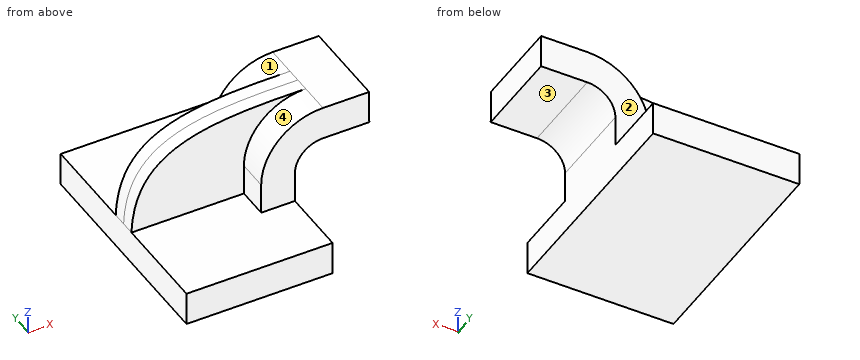
```python
from build123d import *

# Parameters (mm, degrees)
F1_DEPTH = 63.5
F2_DEPTH = 25.4
F3_DEPTH = 7.9375


with BuildPart() as f1:
    # F0 (on Front) → F1 (new body, symmetric)
    with BuildSketch(Plane.XZ):
        Polygon((22.225, 9.525), (-41.275, 9.525), (-41.275, -9.525), (41.275, -9.525), (41.275, 9.525), align=None)
    extrude(amount=F1_DEPTH, both=True)

    # F0 (on Front) → F2 (join, symmetric)
    with BuildSketch(Plane.XZ):
        with BuildLine():
            Line((22.225, 27.0002), (22.225, 9.525))
            Line((22.225, 9.525), (41.275, 9.525))
            Line((41.275, 9.525), (41.275, 27.0002))
            ThreePointArc((41.275, 27.0002), (45.9246798487, 38.2255201513), (57.15, 42.8752))
            Line((57.15, 42.8752), (60.325, 42.8752))
            Line((60.325, 42.8752), (60.325, 61.9252))
            Line((60.325, 61.9252), (57.15, 61.9252))
            ThreePointArc((57.15, 61.9252), (32.4542956671, 51.6959043329), (22.225, 27.0002))
        make_face()
        Polygon((83.2245436112, 61.9252), (60.325, 61.9252), (60.325, 42.8752), (83.2786646287, 42.8752), align=None)
    extrude(amount=F2_DEPTH, both=True)

    # F0 (on Front) → F3 (join, symmetric)
    with BuildSketch(Plane.XZ):
        with BuildLine():
            add(Edge.make_bspline(
                [(57.15, 61.9252), (0, 62.4593123794), (-39.5135097206, 58.9755401015), (-41.275, 9.525)],
                knots=[0, 0, 0, 0, 111.5045361635, 111.5045361635, 111.5045361635, 111.5045361635], degree=3))
            Line((-41.275, 9.525), (22.225, 9.525))
            Line((22.225, 9.525), (22.225, 27.0002))
            ThreePointArc((22.225, 27.0002), (32.4542956671, 51.6959043329), (57.15, 61.9252))
        make_face()
    extrude(amount=F3_DEPTH, both=True)


solid = f1.part
```
The model under review builds one solid part; all positions refer to its coordinate system, in mm. Face numbers are marked on the shaded views. A direction names the side the tool comes from. Round coordinates to 2 decimals unless told otherwise and drop trailing zeros. Loops run counter-clockwise (first coordinate to the right, second up) from the corner with the lowest first, then second, coordinate; pieces in that order, holes last. Notation, with made-up numbers: M -34.75,78.5 L 3.25,78.5 A14 cw 3.25,103.5 Z; hole C 34.5,-17 d8. An arc over 180 degrees is marked long. Put each result on its own line as item: value.
Q1. To check wall thickness, follow L1, parallel to Z at x = 20, y = 53 (3 decimals); L2, parallel to X at y = 19, z = 26.5 (3 decimals); L3, parallel to Z at x = 64.5, y = -4. State the ranges of each line that lie inside material, in increasing order.
Result set:
L1: z = -9.525 to 9.525
L2: x = 22.225 to 41.275
L3: z = 42.88 to 61.93
Q2. Consider section B-B, the plane x = 69.5. Give the boundary of the cut face in (y, z), then the cut area to 3 significant figures.
Result set:
outline: M -25.4,42.88 L 25.4,42.88 L 25.4,61.93 L -25.4,61.93 Z
area: 968 mm²
Q3. Machinability: for the marked faces 1, 2, 3 and 4, which of the approach directions +Z, -Z, +X, -X, +Y, -Y give a long, thin tool a straight path to every point of the face, cutting with its end or side? Answer none if there is none.
Result set:
face 1: +Z, -X, +Y
face 2: +Z, +X, -X, +Y
face 3: -Z, +X, +Y, -Y
face 4: +Z, -X, -Y
Q4. Consider section A-A, the plane y = 10. Give the boundary of the cut face in (x, z) (3 decimals).
Result set:
outline: M -41.275,-9.525 L 41.275,-9.525 L 41.275,27 A15.875 cw 57.15,42.875 L 83.279,42.875 L 83.225,61.925 L 57.15,61.925 A34.925 ccw 22.225,27 L 22.225,9.525 L -41.275,9.525 Z
Q5. Consider section C-C, the plane z = 5.5. Give the boundary of the cut face in (x, y) (3 decimals).
Result set:
outline: M -41.275,-63.5 L 41.275,-63.5 L 41.275,63.5 L -41.275,63.5 Z
Q6. For pin 1 (8.5 mm diameter, centred on y = -17.5, z = 14, fed in from -X) (3 decimals); pin 2 (16.5 mm diameter, centred on x = -15.5, y = -29.5, fed in from +Z) (3 decimals); pin 3 (8 mm diameter, centred on x = 19, z = 25, fed in from -Y), all flat-tipped, find the tip position at first contact; note any pin that passes through.
Result set:
pin 1: stops at x = 22.225
pin 2: stops at z = 9.525
pin 3: stops at y = -25.4
